from build123d import *


with BuildPart() as part:
    # Sketch1 → Revolve1 (revolve)
    with BuildSketch(Plane(origin=(0, 0, 0), x_dir=(1, 0, 0), z_dir=(0, 1, 0))):
        with BuildLine():
            ThreePointArc((12.5603, 2.032), (12.812582596, 2.122503889), (12.949803492, 2.352738309))
            Line((12.949803492, 2.352738309), (13.3985, 4.6482))
            Line((13.3985, 4.6482), (14.986, 4.6482))
            Line((14.986, 4.6482), (14.986, 3.0607))
            ThreePointArc((14.986, 3.0607), (14.089541725, 0.896458275), (11.9253, 0))
            Line((11.9253, 0), (4.7625, 0))
            Line((4.7625, 0), (4.7625, 2.032))
            Line((4.7625, 2.032), (12.5603, 2.032))
        make_face()
    revolve(axis=Axis((0, 0, 0), (0, 0, -1)))


solid = part.part
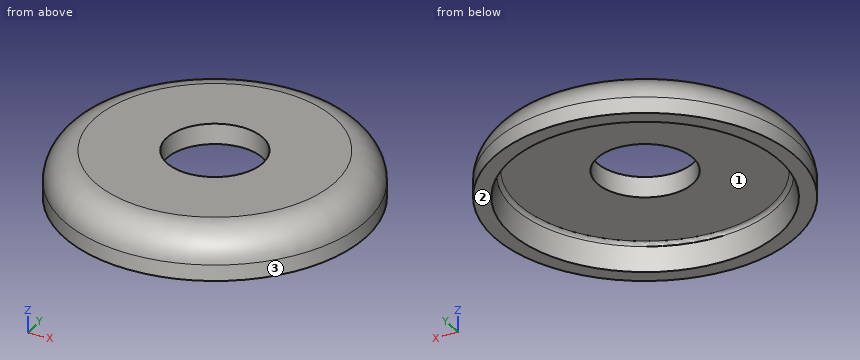
Geometry: final body of the model. Coordinates: model frame, mm. Face numbers are marked on the shaded views. Round coordinates to 2 decimals unless told otherwise and drop trailing zeros. Write each loop counter-clockwise with the first axis right and the second up, starting at its lowest first coordinate (ties: lowest second). Pieces come first, ordered by that corner, then holes. Notation, with made-up numbers: M -5,-5 L 23,-5 A22 ccw 23,34 Z; hole C -32.5,39.5 d3. An arc over 180 degrees is marked long. Write item = value, one per line.
Item 1: Material intervals for line 1 along Z through (x, y) = (8.5, -1.5); line 2 along X through (y, z) = (6, -3.7); line 3 along Y through (x, z) = (-7.5, -3.6), sorted ascending. Write a range as [from, to].
Findings:
line_1 = [-2.03, 0]
line_2 = [-13.73, -11.77], [11.77, 13.73]
line_3 = [-12.97, -10.85], [10.85, 12.97]
Item 2: Pin query (flat end, axial travel): P1, Ø8.5, axis at x = 0, y = 0, coming from the -Z side; P2, Ø1, axis at x = -10.5, y = -4.5, coming from the -Z side; P3, Ø1, axis at y = 1, z = -1, coming from the -X side; P4, Ø1, axis at x = -11.5, z = -3.5, coming from the -Y side. Return the tip coordinate at first contact, or that it passes through.
Findings:
P1 = through
P2 = -2.03
P3 = -14.53
P4 = -10.18
Item 3: Section query C-C on z = -4.2. Return loops of the section in (x, y), then the cut area to 3 significant figures.
Findings:
outline = C 0,0 d29.97; hole C 0,0 d26.62
area = 149 mm^2
Item 4: Section query A-A on x = 0. Return loops of the section in (y, z), then the cut area to 3 significant figures.
Findings:
outline = M -14.99,-4.65 L -13.4,-4.65 L -12.95,-2.35 A0.4 cw -12.56,-2.03 L -4.76,-2.03 L -4.76,0 L -11.93,0 A3.06 ccw -14.99,-3.06 Z; M 4.76,-2.03 L 12.56,-2.03 A0.4 cw 12.95,-2.35 L 13.4,-4.65 L 14.99,-4.65 L 14.99,-3.06 A3.06 ccw 11.93,0 L 4.76,0 Z
area = 47.2 mm^2
Item 5: Pull-direction query (X, two-part tool) for the marked faces 1, 2 and 3; classes: pulls with the +X half, pulls with the -X half, needs draft (parallel to the pull), parting line crosses it, or undercut.
Findings:
face_1 = undercut
face_2 = needs draft
face_3 = parting line crosses it
Item 6: Section query D-D on z = -1.25. Return loops of the section in (x, y) (1 decimal), then the cut area to 3 significant figures.
Findings:
outline = C 0,0 d28.8; hole C 0,0 d9.5
area = 580 mm^2
